The model under review builds one solid part; all positions refer to its coordinate system, in mm. Round coordinates to 2 decimals unless told otherwise and drop trailing zeros. Write each loop counter-clockwise with the first axis right and the second up, starting at its lowest first coordinate (ties: lowest second). Pieces come first, ordered by that corner, then holes. Notation, with made-up numbers: (-19.75, -9.5) -> (6.25, -9.5) arc R25 ccw to (6.25, 23.5) -> close; hole circle Ø6 at (85.25, 47.25). An arc over 180 degrees is marked (long way). Return JSON: item names as keys, results as strings. Group by question number.
1. Take a section at C-C, the plane y = 38.1. Write out the cut boundary in (x, z) (3 decimals).
2. Clearance check with flat-ended pins moving along their axes: P1, Ø1.6, axis at x = 76.2, z = 22.225, coming from the -Y side; P2, Ø3, axis at y = -9.525, z = 22.225, coming from the +X side; P3, Ø10.5, axis at x = 8, y = -6.5, coming from the -Z side (3 decimals); P4, Ø2, axis at x = 23.5, z = 18, coming from the -Y side. State where each tip first meets the part, or that it passes through.
3. Take a section at B-B, the plane z = -2.5. Write out the cut boundary in (x, y) (3 decimals).
4. For line 1 along X through (y, z) = (9.5, 15.5); line 2 along Y through (x, z) = (-63.5, 7) (3 decimals); line 3 along Z through (x, y) = (50.8, 20.5) (3 decimals), list the stretches that pass through material, from the lowest coordinate up. Write a range as from..to.
5. Take a section at A-A, the plane x = 63.5. Write out the cut boundary in (y, z) (3 decimals), then the cut area to 3 significant figures.
6. Take a section at D-D, the plane z = 18. Write out the cut boundary in (x, y) (3 decimals), then the cut area to 3 significant figures.
from build123d import *

# Parameters (mm, degrees)
SKETCH1_W               = 165.1
SKETCH1_H               = 57.15
BOSS_EXTRUDE1_DEPTH     = 47.625
SKETCH6_W               = 9.525
SKETCH6_H               = 19.05
BOSS_EXTRUDE2_DEPTH     = 12.7
F_4_40_TAPPED_HOLE1_D   = 2.2606
F_1_4_20_TAPPED_HOLE1_D = 5.1054
F_6_32_TAPPED_HOLE1_D   = 2.7051


with BuildPart() as part:
    # Sketch1 → Boss-Extrude1 (new body)
    with BuildSketch(Plane(origin=(0, 0, 0), x_dir=(1, 0, 0), z_dir=(0, 1, 0))):
        Rectangle(SKETCH1_W, SKETCH1_H)
    extrude(amount=BOSS_EXTRUDE1_DEPTH)

    # Sketch6 → Boss-Extrude2 (add)
    with BuildSketch(Plane.XY.offset(28.575)):
        with Locations((7.9375, -9.525)):
            Rectangle(SKETCH6_W, SKETCH6_H)
    extrude(amount=-BOSS_EXTRUDE2_DEPTH)

    # #4-40 Tapped Hole1 (through all)
    with Locations(Plane(origin=(12.7, 0, 0), x_dir=(0, 0, -1), z_dir=(1, 0, 0))):
        with Locations((-22.225, -9.525)):
            Hole(F_4_40_TAPPED_HOLE1_D / 2)

    # 1/4-20 Tapped Hole1 (through all)
    with Locations(Plane.XY.offset(28.575)):
        with Locations((-63.5, 38.1), (-63.5, 9.525), (63.5, 38.1), (63.5, 9.525)):
            Hole(F_1_4_20_TAPPED_HOLE1_D / 2)

    # #6-32 Tapped Hole1 (through all)
    with Locations(Plane(origin=(0, 47.625, 0), x_dir=(1, 0, 0), z_dir=(0, 1, 0))):
        with Locations((-76.2, -22.225), (-50.8, -22.225), (50.8, -22.225), (76.2, -22.225)):
            Hole(F_6_32_TAPPED_HOLE1_D / 2)


solid = part.part
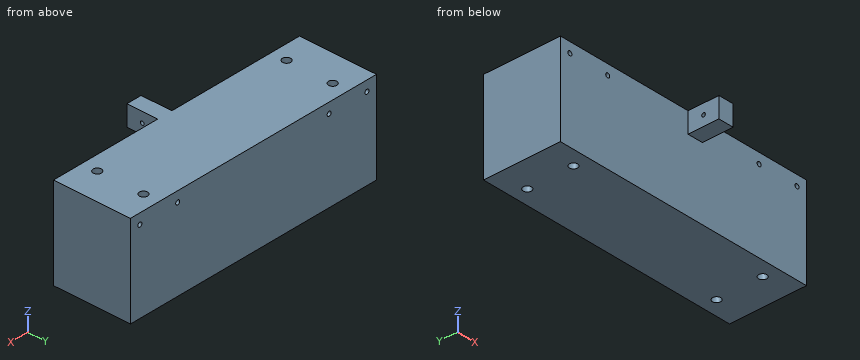
Output:
{
 "1": {"outline": "(-82.55, -28.575) -> (-66.053, -28.575) -> (-66.053, 28.575) -> (-82.55, 28.575) -> close; (-60.947, -28.575) -> (60.947, -28.575) -> (60.947, 28.575) -> (-60.947, 28.575) -> close; (66.053, -28.575) -> (82.55, -28.575) -> (82.55, 28.575) -> (66.053, 28.575) -> close; hole circle Ø2.705 at (-76.2, 22.225); hole circle Ø2.705 at (-50.8, 22.225); hole circle Ø2.705 at (50.8, 22.225); hole circle Ø2.705 at (76.2, 22.225)"},
 "2": {"P1": "passes through", "P2": "stops at x = 12.7", "P3": "stops at z = 15.875", "P4": "stops at y = 0"},
 "3": {"outline": "(-82.55, 0) -> (82.55, 0) -> (82.55, 47.625) -> (-82.55, 47.625) -> close; hole circle Ø5.105 at (-63.5, 9.525); hole circle Ø5.105 at (-63.5, 38.1); hole circle Ø5.105 at (63.5, 9.525); hole circle Ø5.105 at (63.5, 38.1)"},
 "4": {"line 1": "x = -82.55..-66.05, -60.95..60.95, 66.05..82.55", "line 2": "y = 0..6.972, 12.078..35.547, 40.653..47.625", "line 3": "z = -28.575..20.872, 23.578..28.575"},
 "5": {"outline": "(0, -28.575) -> (6.972, -28.575) -> (6.972, 28.575) -> (0, 28.575) -> close; (12.078, -28.575) -> (35.547, -28.575) -> (35.547, 28.575) -> (12.078, 28.575) -> close; (40.653, -28.575) -> (47.625, -28.575) -> (47.625, 28.575) -> (40.653, 28.575) -> close", "area": "2,140 mm^2"},
 "6": {"outline": "(-82.55, 0) -> (3.175, 0) -> (3.175, -19.05) -> (12.7, -19.05) -> (12.7, 0) -> (82.55, 0) -> (82.55, 47.625) -> (-82.55, 47.625) -> close; hole circle Ø5.105 at (-63.5, 9.525); hole circle Ø5.105 at (-63.5, 38.1); hole circle Ø5.105 at (63.5, 9.525); hole circle Ø5.105 at (63.5, 38.1)", "area": "7,960 mm^2"}
}
